Check sheet for the modelled part. Datum: model origin and axes. Units: mm. Face numbers are marked on the shaded views. A direction names the side the tool comes from. Give positions to 0.01 mm unless a question says otherwise; leave off trailing zeros. Loops run counter-clockwise (first coordinate to the right, second up) from the corner with the lowest first, then second, coordinate; pieces in that order, holes last. Notation, with made-up numbers: (15, 86.5) -> (59, 86.5) arc R7 cw to (59, 99.5) -> close; hole circle Ø10 at (12.5, 81). An arc over 180 degrees is marked (long way). Write each question's results on one line, items separated by ' | '. Start each with the question number.
Item 1: Gauge pin test, flat end, axial feed: pin 1 Ø2 at (x, z) = (-7.5, -3) entering from +Y. Record the tip position at first contact, or that the pin passes through.
Item 2: Cross-section at C-C on z = -3. State how many separate pieces and enclosed holes the cut face has, then the cut area to 3 significant figures.
Item 3: Cross-section at A-A on y = 0. Enter the section's corners in (x, z).
Item 4: Mould release check, pull along X, two halves, no side actions. Record for the marked faces 1, 2, 3 and 4: pulls with the +X half, pulls with the -X half, needs draft (parallel to the pull), parting line crosses it, or undercut.
Item 5: Cross-section at B-B on y = 20. Enter the section's corners in (x, z).
Item 6: Access from +Z, -Z, +X, -X, +Y, -Y to the whole of each face (thin tool, end or side, straight path). Record for the marked faces 5, 6, 7, 8 and 9.
Item 7: Scan lines: line 1 along X through (y, z) = (-7, -0.15); line 2 along Y through (x, z) = (19, -1.5); line 3 along Y through (x, z) = (18.5, -2.45). Record each from-to range of solid material in increasing order.
from build123d import *

# Parameters (mm, degrees)
CROQUIS7_R              = 11
CROQUIS7_R_2            = 1
SALIENTE_EXTRUIR4_DEPTH = 4
CORTAR_EXTRUIR3_DEPTH   = 17.062378404
MATRIZC3_COUNT          = 20
CROQUIS9_R              = 1
CROQUIS9_R_2            = 1.25
SALIENTE_EXTRUIR5_DEPTH = 4
CROQUIS2_R              = 1
CROQUIS2_R_2            = 1.5
SALIENTE_EXTRUIR2_DEPTH = 4
CORTAR_EXTRUIR4_DEPTH   = 33.078029865
CHAFL_N1_SIZE           = 0.5


with BuildPart() as part:
    # Croquis7 → Saliente-Extruir4 (new body)
    with BuildSketch(Plane.XY):
        Circle(CROQUIS7_R)
        Circle(CROQUIS7_R_2, mode=Mode.SUBTRACT)
    extrude(amount=-SALIENTE_EXTRUIR4_DEPTH)

    # Croquis10 → Cortar-Extruir3 (cut, through all)
    with BuildSketch(Plane.XY):
        with BuildLine():
            ThreePointArc((0.499924007, 8.734705318), (0, 8.749), (-0.499924007, 8.734705318))
            ThreePointArc((-0.499924007, 8.734705318), (-0.824302243, 9.905497836), (-1.485192705, 10.924909509))
            ThreePointArc((-1.485192705, 10.924909509), (0, 11.0254), (1.485192705, 10.924909509))
            ThreePointArc((1.485192705, 10.924909509), (0.824302243, 9.905497836), (0.499924007, 8.734705318))
        make_face()
    cortar_extruir3 = extrude(amount=-CORTAR_EXTRUIR3_DEPTH, mode=Mode.SUBTRACT)

    # MatrizC3: Cortar-Extruir3 ×20 about axis
    matrizc3_axis = Axis((0, 0, 0), (0, 0, 1))
    for i in range(1, MATRIZC3_COUNT):
        add(cortar_extruir3.rotate(matrizc3_axis, i * 360 / MATRIZC3_COUNT), mode=Mode.SUBTRACT)

    # Croquis9 → Saliente-Extruir5 (add)
    with BuildSketch(Plane.XY):
        with BuildLine():
            Line((0.210526316, 3.994455992), (19.157894737, 2.995841994))
            ThreePointArc((19.157894737, 2.995841994), (22, 0), (19.157894737, -2.995841994))
            Line((19.157894737, -2.995841994), (0.210526316, -3.994455992))
            ThreePointArc((0.210526316, -3.994455992), (-4, 0), (0.210526316, 3.994455992))
        make_face()
        Circle(CROQUIS9_R, mode=Mode.SUBTRACT)
        with Locations((19, 0)):
            Circle(CROQUIS9_R_2, mode=Mode.SUBTRACT)
    extrude(amount=-SALIENTE_EXTRUIR5_DEPTH)

    # Croquis2 → Saliente-Extruir2 (add, through all)
    with BuildSketch(Plane.XY.offset(-4)):
        with BuildLine():
            Line((-3.171102714, 20.998669186), (3.771863049, 1.331558915))
            ThreePointArc((3.771863049, 1.331558915), (1.149391542, -3.831305141), (-3.881954792, -0.964586438))
            Line((-3.881954792, -0.964586438), (-8.911466094, 19.276560172))
            ThreePointArc((-8.911466094, 19.276560172), (-6.862043657, 22.873478856), (-3.171102714, 20.998669186))
        make_face()
        Circle(CROQUIS2_R, mode=Mode.SUBTRACT)
        with Locations((-6, 20)):
            Circle(CROQUIS2_R_2, mode=Mode.SUBTRACT)
    extrude(amount=SALIENTE_EXTRUIR2_DEPTH)

    # Croquis11 → Cortar-Extruir4 (cut, through all)
    with BuildSketch(Plane(origin=(0, 0, -4), x_dir=(-1, 0, 0), z_dir=(0, 0, -1))):
        with BuildLine():
            Line((-0.780626911, 9.804734929), (-1.788639616, 6.949370564))
            ThreePointArc((-1.788639616, 6.949370564), (-3.478211644, 4.651731754), (-6.159867825, 3.680898163))
            Line((-6.159867825, 3.680898163), (-8.789028829, 3.542329211))
            Line((-8.789028829, 3.542329211), (-14.154797023, 5.193302426))
            Line((-14.154797023, 5.193302426), (-17.039697184, 17.319662426))
            Line((-17.039697184, 17.319662426), (-0.365952184, 17.319662426))
            Line((-0.365952184, 17.319662426), (-0.780626911, 9.804734929))
        make_face()
    extrude(amount=-CORTAR_EXTRUIR4_DEPTH, mode=Mode.SUBTRACT)

    # Chaflán1
    chafl_n1_edges = [part.edges().sort_by_distance(p)[0] for p in [
        (13.973461783, -3.269085602, -4),
        (12.658881281, 3.338370078, -4),
        (22, 0, -4),
        (13.973461783, -3.269085602, 0),
        (22, 0, 0),
        (12.658881281, 3.338370078, 0),
        (-0.691231549, 13.974019875, -4),
        (-7.399550596, 13.191892812, -4),
        (-0.691231549, 13.974019875, 0),
        (-6.862043657, 22.873478856, 0),
        (-7.399550596, 13.191892812, 0),
        (-6.862043657, 22.873478856, -4),
        (3.478211644, 4.651731754, -4),
        (3.478211644, 4.651731754, 0),
    ]]
    chamfer(chafl_n1_edges, length=CHAFL_N1_SIZE)


solid = part.part
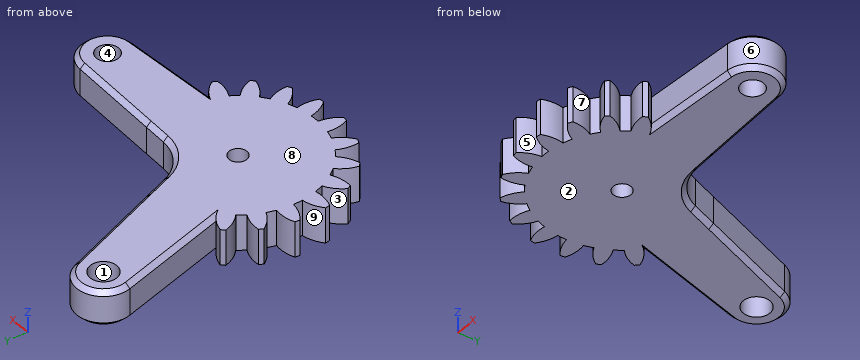
Answer sheet:
1) pin 1: stops at y = 22.96
2) separate pieces: 1 | enclosed holes: 3 | area: 425 mm²
3) outline: (-8.75, -4) -> (-1, -4) -> (-1, 0) -> (-8.75, 0) -> close; (1, -4) -> (17.75, -4) -> (17.75, 0) -> (1, 0) -> close; (20.25, -4) -> (21.5, -4) -> (22, -3.5) -> (22, -0.5) -> (21.5, 0) -> (20.25, 0) -> close
4) face 1: undercut | face 2: needs draft | face 3: pulls with the -X half | face 4: undercut
5) outline: (-9, -3.5) -> (-8.5, -4) -> (-7.5, -4) -> (-7.5, 0) -> (-8.5, 0) -> (-9, -0.5) -> close; (-4.5, -4) -> (-3.35, -4) -> (-2.82, -3.5) -> (-2.82, -0.5) -> (-3.35, 0) -> (-4.5, 0) -> close
6) face 5: +Z, -Z, -Y | face 6: +Z, -Z, +X | face 7: +Z, -Z | face 8: +Z, +X, -X, +Y, -Y | face 9: +Z, -Z, -X
7) line 1: x = -7.78 to -5.77, -5.25 to 5.25, 5.77 to 7.78 | line 2: y = -3 to -1.25, 1.25 to 3 | line 3: y = -3.03 to -1.15, 1.15 to 3.03
